Geometry: final body of the model. Coordinates: model frame, mm. Coordinates: 2 decimals unless noted, no trailing zeros. Write each loop counter-clockwise with the first axis right and the second up, starting at its lowest first coordinate (ties: lowest second). Pieces come first, ordered by that corner, then holes. Notation, with made-up numbers: (53.25, 53) -> (57.25, 53) arc R16 cw to (57.25, 84) -> close; hole circle Ø7 at (20.5, -0.75). An arc over 180 degrees is marked (long way). Answer as a JSON object with one key per item and string values. Group by question number.
```python
from build123d import *

# Parameters (mm, degrees)
F0_W     = 159.9906936405
F0_H     = 160
F2_DEPTH = 6.35
F3_DEPTH = 6.351
F4_DEPTH = 25
F5_DEPTH = 25
F6_DEPTH = 25
F7_DEPTH = 25


with BuildPart() as f2:
    # F0 (on Top) → F2 (new body)
    with BuildSketch(Plane.XY):
        Rectangle(F0_W, F0_H)
    extrude(amount=-F2_DEPTH)

    # F1 (on face) → F3 (cut, through all)
    with BuildSketch(Plane.XY):
        with BuildLine():
            add(Edge.make_bspline(
                [(-8.1994745377, 24.4279390933), (-19.7248762604, 35.8088584368), (-26.0936386648, 19.0302092428), (-32.4624010693, 2.2515600487), (-15.2297855146, 5.9064251608)],
                knots=[0, 0, 0, 2.0353938469, 2.0353938469, 4.0707876938, 4.0707876938, 4.0707876938], degree=2, weights=[1, 0.5253270315, 1, 0.5253270315, 1]))
            ThreePointArc((-15.2297855146, 5.9064251608), (-11.4929489268, 11.6079433995), (-5.7545107942, 15.2878327607))
            add(Edge.make_bspline(
                [(-5.7545107942, 15.2878327607), (-4.5186333902, 20.7932409522), (-8.1994745377, 24.4279390933)],
                knots=[5.3284067292, 5.3284067292, 5.3284067292, 6.2831853072, 6.2831853072, 6.2831853072], degree=2, weights=[1, 0.8881974706, 1]))
        make_face()
    extrude(amount=-F3_DEPTH, mode=Mode.SUBTRACT)

    # F1 (on face) → F4 (cut)
    with BuildSketch(Plane.XY):
        with BuildLine():
            add(Edge.make_bspline(
                [(5.7545107942, 15.2878327607), (7.4920907008, 7.5475127097), (15.2297855146, 5.9064251608)],
                knots=[0.954778578, 0.954778578, 0.954778578, 2.2123976134, 2.2123976134, 2.2123976134], degree=2, weights=[1, 0.808728302, 1]))
            ThreePointArc((15.2297855146, 5.9064251608), (11.4929489268, 11.6079433995), (5.7545107942, 15.2878327607))
        make_face()
    extrude(amount=-F4_DEPTH, mode=Mode.SUBTRACT)

    # F1 (on face) → F5 (cut)
    with BuildSketch(Plane.XY):
        with BuildLine():
            ThreePointArc((5.7545107942, 15.2878327607), (11.4929489268, 11.6079433995), (15.2297855146, 5.9064251608))
            add(Edge.make_bspline(
                [(15.2297855146, 5.9064251608), (32.4624010693, 2.2515600487), (26.0936386648, 19.0302092428), (19.7248762604, 35.8088584368), (8.1994745377, 24.4279390933)],
                knots=[2.2123976134, 2.2123976134, 2.2123976134, 4.2477914603, 4.2477914603, 6.2831853072, 6.2831853072, 6.2831853072], degree=2, weights=[1, 0.5253270315, 1, 0.5253270315, 1]))
            add(Edge.make_bspline(
                [(8.1994745377, 24.4279390933), (4.5186333902, 20.7932409522), (5.7545107942, 15.2878327607)],
                knots=[0, 0, 0, 0.954778578, 0.954778578, 0.954778578], degree=2, weights=[1, 0.8881974706, 1]))
        make_face()
    extrude(amount=-F5_DEPTH, mode=Mode.SUBTRACT)

    # F1 (on face) → F6 (cut)
    with BuildSketch(Plane.XY):
        with BuildLine():
            ThreePointArc((-5.7545107942, 15.2878327607), (-11.4929489268, 11.6079433995), (-15.2297855146, 5.9064251608))
            add(Edge.make_bspline(
                [(-15.2297855146, 5.9064251608), (-7.4920907008, 7.5475127097), (-5.7545107942, 15.2878327607)],
                knots=[4.0707876938, 4.0707876938, 4.0707876938, 5.3284067292, 5.3284067292, 5.3284067292], degree=2, weights=[1, 0.808728302, 1]))
        make_face()
    extrude(amount=-F6_DEPTH, mode=Mode.SUBTRACT)

    # F1 (on face) → F7 (cut)
    with BuildSketch(Plane.XY):
        with BuildLine():
            ThreePointArc((-15.2297855146, 5.9064251608), (-3.0044698883, -16.0563191825), (16.335, 0))
            ThreePointArc((16.335, 0), (16.0563191825, 3.0044698883), (15.2297855146, 5.9064251608))
            add(Edge.make_bspline(
                [(5.7545107942, 15.2878327607), (7.4920907008, 7.5475127097), (15.2297855146, 5.9064251608)],
                knots=[0.954778578, 0.954778578, 0.954778578, 2.2123976134, 2.2123976134, 2.2123976134], degree=2, weights=[1, 0.808728302, 1]))
            ThreePointArc((5.7545107942, 15.2878327607), (0, 16.335), (-5.7545107942, 15.2878327607))
            add(Edge.make_bspline(
                [(-15.2297855146, 5.9064251608), (-7.4920907008, 7.5475127097), (-5.7545107942, 15.2878327607)],
                knots=[4.0707876938, 4.0707876938, 4.0707876938, 5.3284067292, 5.3284067292, 5.3284067292], degree=2, weights=[1, 0.808728302, 1]))
        make_face()
    extrude(amount=-F7_DEPTH, mode=Mode.SUBTRACT)


solid = f2.part
```
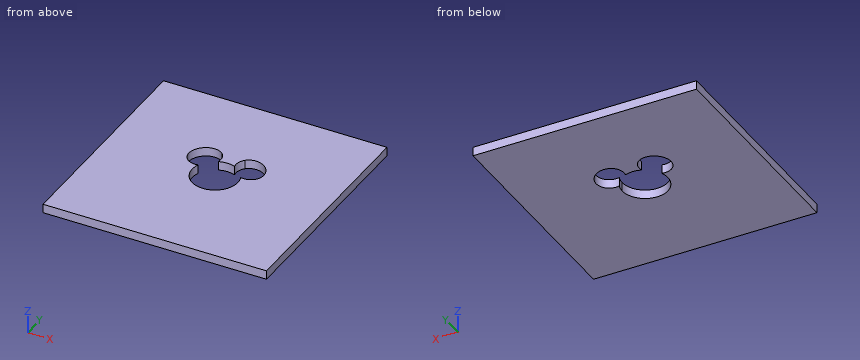
Item 1: Section A-A on x = 0. Output: boundary loops of the cut face in (y, z) (3 decimals), then the cut area to 3 significant figures.
Item 2: Ray query, L1, parallel to X at y = 0, z = -2 (3 decimals); L2, parallel to Y at x = 0, z = -4.25 (3 decimals); L3, parallel to Y at x = 24.5, z = -3.5. Return the intervals inside material, ascending. Write a range as [from, to].
Item 3: Section B-B on y = 19.5. Give the number of separate pieces and of enclosed holes in the cut face, then the cut area to 3 significant figures.
Answer sheet:
{
 "1": {"outline": "(-80, -6.35) -> (-16.335, -6.35) -> (-16.335, 0) -> (-80, 0) -> close; (16.335, -6.35) -> (80, -6.35) -> (80, 0) -> (16.335, 0) -> close", "area": "809 mm^2"},
 "2": {"L1": "x = [-79.995, -16.335], [16.335, 79.995]", "L2": "y = [-80, -16.335], [16.335, 80]", "L3": "y = [-80, 8.69], [21.96, 80]"},
 "3": {"separate pieces": "3", "enclosed holes": "0", "area": "759 mm^2"}
}
